from build123d import *

# Parameters (mm, degrees)
F0_W      = 112
F0_H      = 56
F1_DEPTH  = 17
F3_R      = 12.5
F4_DEPTH  = 17
F6_R      = 28
F7_DEPTH  = 13
F8_DEPTH  = 25
F10_R     = 4
F11_DEPTH = 28.001
F12_R     = 5
F13_DEPTH = 17.001
F16_DEPTH = 6
F18_DEPTH = 56.5010001


with BuildPart() as f1:
    # F0 (on Top) → F1 (new body)
    with BuildSketch(Plane.XY):
        Rectangle(F0_W, F0_H)
    extrude(amount=F1_DEPTH)

    # F3 (on offset) → F4 (join)
    with BuildSketch(Plane(origin=(0, 24, 0), x_dir=(-1, 0, 0), z_dir=(0, 1, 0))):
        with BuildLine():
            Line((-26.4197592234, 101.2734202201), (-56, 17))
            Line((-56, 17), (56, 17))
            Line((56, 17), (26.4197592234, 101.2734202201))
            ThreePointArc((26.4197592234, 101.2734202201), (27.6021127656, 96.7035487531), (28, 92))
            ThreePointArc((28, 92), (-4.7035487531, 64.3978872344), (-26.4197592234, 101.2734202201))
        make_face()
        with BuildLine():
            ThreePointArc((26.4197592234, 101.2734202201), (0, 120), (-26.4197592234, 101.2734202201))
            ThreePointArc((-26.4197592234, 101.2734202201), (-4.7035487531, 64.3978872344), (28, 92))
            ThreePointArc((28, 92), (27.6021127656, 96.7035487531), (26.4197592234, 101.2734202201))
        make_face()
        with Locations((0, 92)):
            Circle(F3_R, mode=Mode.SUBTRACT)
    extrude(amount=-F4_DEPTH)

    # F6 (on offset) → F7 (join, symmetric)
    with BuildSketch(Plane(origin=(0, 15.5, 0), x_dir=(-1, 0, 0), z_dir=(0, 1, 0))):
        with Locations((0, 92)):
            Circle(F6_R)
    extrude(amount=F7_DEPTH, both=True)

    # F3 (on offset) → F8 (cut, symmetric)
    with BuildSketch(Plane(origin=(0, 24, 0), x_dir=(-1, 0, 0), z_dir=(0, 1, 0))):
        with Locations((0, 92)):
            Circle(F3_R)
    extrude(amount=F8_DEPTH, both=True, mode=Mode.SUBTRACT)

    # F10 (on offset) → F11 (cut, through all)
    with BuildSketch(Plane.XY.offset(92)):
        with Locations((0, 15.5)):
            Circle(F10_R)
    extrude(amount=F11_DEPTH, mode=Mode.SUBTRACT)

    # F12 (on face) → F13 (cut, through all)
    with BuildSketch(Plane.XY.offset(17)):
        with Locations((-44, -10)):
            Circle(F12_R)
        with Locations((44, -10)):
            Circle(F12_R)
    extrude(amount=-F13_DEPTH, mode=Mode.SUBTRACT)

    # F15 (on offset) → F16 (join, symmetric)
    with BuildSketch(Plane.YZ):
        Polygon((7, 17), (7, 49), (-28, 17), align=None)
    extrude(amount=F16_DEPTH, both=True)

    # F17 (on face) → F18 (cut, through all)
    with BuildSketch(Plane.XZ.offset(28)):
        with BuildLine():
            Line((31, 3), (-31, 3))
            ThreePointArc((-31, 3), (-34, 0), (-31, -3))
            Line((-31, -3), (31, -3))
            ThreePointArc((31, -3), (34, 0), (31, 3))
        make_face()
    extrude(amount=-F18_DEPTH, mode=Mode.SUBTRACT)


solid = f1.part
Build history of the part. All positions in model axes, mm. A direction names the side the tool comes from. Coordinates: 2 decimals unless noted, no trailing zeros. Write each loop counter-clockwise with the first axis right and the second up, starting at its lowest first coordinate (ties: lowest second). Pieces come first, ordered by that corner, then holes.
(1) 3-axis set-ups, long thin cutter, end or side, ignore diameter. For faces 1 (the flat face through (-1, 26, 17)), 2 (the flat face through (-6, -3, 26)), 3 (the flat face through (0, 0, 3)), 4 (the flat face through (1, 7, 50)), 5 (the flat face through (-1, 28, 8)): which of +Z, -Z, +X, -X, +Y, -Y reach the whole face in a straight line?
(2) Pin check, flat tips, straight feed: pin 1 Ø8 at (x, z) = (36.5, 32.5) entering from -Y; pin 2 Ø17 at (x, z) = (12.5, 83.5) entering from -Y; pin 3 Ø8 at (x, y) = (-44, -10) entering from +Z (3 decimals); pin 4 Ø1.5 at (x, y) = (4.5, 13) entering from -Z. Stop position of each tip, or through.
(3) Cut at C-C on x = 44. List the corners of the cut face in (y, z), and give its area (3 significant figures).
(4) Cut at B-B on y = 4. List the corners of the cut face in (x, z).
(5) Drill centre lines: line 1 (Y direction, x = 44, z = 9); line 2 (X direction, y = -11.5, z = 14.5); line 3 (Z direction, x = 29, y = -4). Where is each one in solid material? Low to high.
(6) Mould opens along Y. For faces 6 (the flat face through (-56, 0, 8)), 7 (the flat face through (-6, 2.5, 80)), 8 (the cylindrical face through (-49, -10, 9)) say: pulls with the +Y half, pulls with the -Y half, needs draft (parallel to the pull), parting line crosses it, or undercut.
(7) Cut at A-A on x = 0. List the corners of the cut face in (y, z).
(8) Cut at D-D on y = -10. List the corners of the cut face in (x, z).
Working result:
1. face 1: +X, -X, +Y
1. face 2: -X, -Y
1. face 3: -Z, +Y, -Y
1. face 4: -Y
1. face 5: -Z, +X, -X, +Y
2. pin 1: stops at y = 7
2. pin 2: stops at y = 2.5
2. pin 3: passes through
2. pin 4: stops at z = 3
3. outline: (-28, 0) - (-15, 0) - (-15, 17) - (-28, 17) - close; (-5, 0) - (28, 0) - (28, 17) - (24, 17) - (24, 51.19) - (7, 51.19) - (7, 17) - (-5, 17) - close
3. area: 1,360 mm2
4. outline: (-56, 0) - (-34, 0) arc R3 cw to (-31, 3) - (31, 3) arc R3 cw to (34, 0) - (56, 0) - (56, 17) - (6, 17) - (6, 46.26) - (-6, 46.26) - (-6, 17) - (-56, 17) - close; circle Ø56 at (0, 92); hole circle Ø25 at (0, 92)
5. line 1: y = -28 to -15, -5 to 28
5. line 2: x = -56 to -48.77, -39.23 to 39.23, 48.77 to 56
5. line 3: z = 3 to 17
6. face 6: needs draft
6. face 7: pulls with the -Y half
6. face 8: undercut
7. outline: (-28, 3) - (28, 3) - (28, 17) - (24, 17) - (24, 64) - (28.5, 64) - (28.5, 79.5) - (2.5, 79.5) - (2.5, 64) - (7, 64) - (7, 49) - (-28, 17) - close; (2.5, 104.5) - (11.5, 104.5) - (11.5, 120) - (2.5, 120) - close; (19.5, 104.5) - (28.5, 104.5) - (28.5, 120) - (19.5, 120) - close
8. outline: (-56, 0) - (-49, 0) - (-49, 17) - (-56, 17) - close; (-39, 0) - (-34, 0) arc R3 cw to (-31, 3) - (31, 3) arc R3 cw to (34, 0) - (39, 0) - (39, 17) - (6, 17) - (6, 33.46) - (-6, 33.46) - (-6, 17) - (-39, 17) - close; (49, 0) - (56, 0) - (56, 17) - (49, 17) - close
